Here's how the part is built. I have some questions about the finished solid (model axes, mm). A direction names the side the tool comes from. Coordinates: 2 decimals unless noted, no trailing zeros. Loops run counter-clockwise (first coordinate to the right, second up) from the corner with the lowest first, then second, coordinate; pieces in that order, holes last.
```python
from build123d import *

# Parameters (mm, degrees)
SKETCH1_R           = 1.75
BOSS_EXTRUDE1_DEPTH = 1.5
CHAMFER1_SIZE       = 1


with BuildPart() as part:
    # Sketch1 → Boss-Extrude1 (new body)
    with BuildSketch(Plane(origin=(0, 0, 0), x_dir=(1, 0, 0), z_dir=(0, 1, 0))):
        Polygon((0, 0), (29.5, 0), (29.5, -13), (-13, -13), (-13, 29.5), (0, 29.5), align=None)
        with Locations(Location((-6.5, 7.375, 0), (0, 0, 270))):
            Circle(SKETCH1_R, mode=Mode.SUBTRACT)
        with Locations(Location((7.375, -6.5, 0), (0, 0, 270))):
            Circle(SKETCH1_R, mode=Mode.SUBTRACT)
        with Locations(Location((-6.5, 22.125, 0), (0, 0, 90))):
            Circle(SKETCH1_R, mode=Mode.SUBTRACT)
        with Locations(Location((22.125, -6.5, 0), (0, 0, 90))):
            Circle(SKETCH1_R, mode=Mode.SUBTRACT)
    extrude(amount=BOSS_EXTRUDE1_DEPTH)

    # Chamfer1
    chamfer1_edges = [part.edges().sort_by_distance(p)[0] for p in [
        (-6.5, 1.5, -9.125),
        (7.375, 1.5, 4.75),
        (-6.5, 1.5, -20.375),
        (22.125, 1.5, 8.25),
    ]]
    chamfer(chamfer1_edges, length=CHAMFER1_SIZE)


solid = part.part
```
1. We'd pull the mould along X, two halves only. Please class faces 1 (the flat face through (-1, 0, -4)), 2 (the flat face through (-13, 1, -8)), 3 (the cylindrical face through (6.31, 0.25, 5.11)): +X half, -X half, draft (parallel to the pull), parting line (faces both ways), or undercut.
2. I need wall thicknesses on line 1 along X through (y, z) = (0.4, 6.5) (3 decimals); line 2 along X through (y, z) = (1.1, 8.5); line 3 along X through (y, z) = (0.2, -14.5). Which ranges of each line are inside material? Lowest first, please.
3. On a 3-axis mill with a long thin cutter (end or side, diameter ignored), from which of +Z, -Z, +X, -X, +Y, -Y can I reach the whole of each face in a straight line? I mean faces 4 (the flat face through (-7, 1, -29.5)), 5 (the flat face through (15, 1, 0)). Say none if no direction works.
4. For pin 1 (5.5 mm diameter, centred on x = 7.375, z = 6.5, fed in from -Y); pin 2 (3 mm diameter, centred on x = -6.5, z = -22.125, fed in from +Y); pin 3 (4.5 mm diameter, centred on x = -6.5, z = -7.375, fed in from +Y), each with a flat end and sliding along its axis, tell me the tip position at first contact or that it passes through.
5. I want a section at B-B (x = -6.5). Please give me the cut outline in (y, z) (3 decimals).
6. I want a section at A-A (z = 6.5). Please give me the cut outline in (x, y) (3 decimals), then the cut area to 4 significant figures.
7. I want a section at D-D (x = 13). Please give me the cut outline in (y, z), then the cut area to 3 significant figures.
8. I want a section at C-C (y = 1.15). Please give me the cut outline in (x, z) (3 decimals).
Response values:
1. face 1: draft
1. face 2: -X half
1. face 3: undercut
2. line 1: x = -13 to 5.625, 9.125 to 20.375, 23.875 to 29.5
2. line 2: x = -13 to 6.14, 8.61 to 20.89, 23.36 to 29.5
2. line 3: x = -13 to 0
3. face 4: -Z, +X, -X, +Y, -Y
3. face 5: -Z, +X, +Y, -Y
4. pin 1: stops at y = 0
4. pin 2: passes through
4. pin 3: stops at y = 1
5. outline: (0, -29.5) - (1.5, -29.5) - (1.5, -24.875) - (0.5, -23.875) - (0, -23.875) - close; (0, -20.375) - (0.5, -20.375) - (1.5, -19.375) - (1.5, -10.125) - (0.5, -9.125) - (0, -9.125) - close; (0, -5.625) - (0.5, -5.625) - (1.5, -4.625) - (1.5, 13) - (0, 13) - close
6. outline: (-13, 0) - (5.625, 0) - (5.625, 0.5) - (4.625, 1.5) - (-13, 1.5) - close; (9.125, 0) - (20.375, 0) - (20.375, 0.5) - (19.375, 1.5) - (10.125, 1.5) - (9.125, 0.5) - close; (23.875, 0) - (29.5, 0) - (29.5, 1.5) - (24.875, 1.5) - (23.875, 0.5) - close
6. area: 51.25 mm2
7. outline: (0, 0) - (1.5, 0) - (1.5, 13) - (0, 13) - close
7. area: 19.5 mm2
8. outline: (-13, -29.5) - (0, -29.5) - (0, 0) - (29.5, 0) - (29.5, 13) - (-13, 13) - close; hole circle Ø4.8 at (-6.5, -22.125); hole circle Ø4.8 at (-6.5, -7.375); hole circle Ø4.8 at (7.375, 6.5); hole circle Ø4.8 at (22.125, 6.5)
